Check sheet for the modelled part. Datum: model origin and axes. Units: mm. A direction names the side the tool comes from. Round coordinates to 2 decimals unless told otherwise and drop trailing zeros. Write each loop counter-clockwise with the first axis right and the second up, starting at its lowest first coordinate (ties: lowest second). Pieces come first, ordered by that corner, then holes.
Item 1: Tool access check on faces 1 (the flat face through (24, -8, 20)), 2 (the cylindrical face through (2.994, 22.804, 1.479)), 3 (the flat face through (-11.77, 30.07, 4.93)), 4 (the flat face through (-20.16, 25.23, 4.93)). Record the directions out of +Z, -Z, +X, -X, +Y, -Y that give a thin tool (end or side, any length) a straight path to the whole face; none if there is none.
Item 2: Release check for a two-part mould opening along Z. For faces 5 (the cylindrical face through (-26.6, -0.1, 9.5)), 6 (the cylindrical face through (-13.17, -28.36, 15.07)), 7 (the flat face through (33.5, 0.1, 10)) record: +Z half, -Z half, draft (parallel to the pull), parting line (faces both ways), or undercut.
Item 3: Go/stop test with flat-tipped pins: pin 1 Ø2 at (x, y) = (-26, 25) entering from -Z; pin 2 Ø12 at (x, z) = (10.5, 13.5) entering from -Y; pin 3 Ø6 at (y, z) = (-18, 16) entering from +X; pin 4 Ø5 at (y, z) = (-6.5, 15) entering from +X. Record where each tip stops, or that it passes through.
Item 4: Cross-section at D-D on x = -27. Enter the section's corners in (y, z), plus the area to 3 significant figures.
Item 5: Cross-section at B-B on z = 12. Enter the section's corners in (x, y).
Item 6: Cross-section at C-C on y = 0. Count the separate pieces of the cut face and the enclosed holes in it, plus the area to 3 significant figures.
Item 7: Material ranges on line 1 (X direction, y = 0, z = 0.85); line 2 (Y direction, x = 0, z = 13); line 3 (Y direction, x = 0, z = 1.6), recorded low to high.
Autodesk Inventor part; units mm, degrees
ref_plane "Arbeitsebene1" through (-40, 0, 0) normal (1, 0, 0) x (0, 1, 0)
ref_plane "XZ Plane" through (0, 0, 0) normal (0, 1, 0) x (-1, 0, 0)
ref_plane "XY Plane" through (0, 0, 0) normal (0, 0, 1) x (1, 0, 0)
sketch "Skizze1" plane through (0, 0, 0) normal (0, 1, 0) x (-1, 0, 0)
  line L0 (17, 30.75) -> (17, 26.75)
  line L1 (17, 26.75) -> (20, 26.75)
  line L2 (20, 26.75) -> (20, 6.75)
  line L3 (23, 0) -> (35, 0)
  line L4 (35, 0) -> (35, 20)
  line L5 (35, 20) -> (25, 20)
  line L6 (25, 20) -> (25, 30.75)
  line L7 (17, 30.75) -> (25, 30.75)
  line L8 (0, 0) -> (0, 48.4152)
  line L9 (20, 6.75) -> (23, 6.75)
  line L10 (23, 6.75) -> (23, 4.75)
  line L11 (23, 4.75) -> (25, 4.75)
  line L12 (25, 4.75) -> (25, 3)
  line L13 (25, 3) -> (23, 3)
  line L14 (23, 3) -> (23, 0)
  point P0 (17, 4)
  dimension "d1" = 40
  dimension "d3" = 20
  dimension "d4" = 70
  dimension "d5" = 50
  dimension "d7" = 4
  dimension "d10" = 2
  dimension "d11" = 1.75
  dimension "d12" = 3
  dimension "d13" = 3
  dimension "d14" = 2
  dimension "d15" = 34
  dimension "d16" = 20
revolve "Umdrehung1" add sketch "Skizze1" angle 360 about axis through (0, 0, 0) along (0, 0, 1)
sketch "Skizze2" plane through (0, 0, 0) normal (0, 0, -1) x (-1, 0, 0)
  circle A0 centre (0, 0) radius 23
  circle A1 centre (0, 0) radius 35
  arc A2 (-29.325, -4.4491) -> (-29.325, 4.4491) centre (-30, 0) ccw
  line L0 (-29.325, 4.4491) -> (-34.604, 5.25)
  line L1 (-29.325, -4.4491) -> (-34.604, -5.25)
  line L2 (49, 0) -> (-49, 0)
  line L3 (10.8095, -27.6207) -> (12.7554, -32.593)
  arc A3 (18.5155, -23.1717) -> (10.8095, -27.6207) centre (15, -25.9808) ccw
  line L4 (18.5155, -23.1717) -> (21.8486, -27.343)
  line L5 (18.5155, 23.1717) -> (21.8486, 27.343)
  arc A4 (10.8095, 27.6207) -> (18.5155, 23.1717) centre (15, 25.9808) ccw
  line L6 (10.8095, 27.6207) -> (12.7554, 32.593)
  arc A5 (21.8486, 27.343) -> (12.7554, 32.593) centre (0, 0) ccw
  arc A6 (12.7554, -32.593) -> (21.8486, -27.343) centre (0, 0) ccw
  arc A7 (-34.604, 5.25) -> (-34.604, -5.25) centre (0, 0) ccw
  dimension "d17" = 30
  dimension "d18" = 4.5
  dimension "d21" = 360
extrude "Extrusion1" cut sketch "Skizze2" against normal blind 10 contours L2 A1 L0 A2 | A2 L1 A1 L2 | L5 A4 L6 A1 | A1 L3 A3 L4
sketch "Skizze3" plane through (0, 0, 0) normal (0, 0, -1) x (-1, 0, 0)
  arc A0 (10.8095, 27.6207) -> (18.5155, 23.1717) centre (15, 25.9808) ccw
  arc A1 (-29.325, -4.4491) -> (-29.325, 4.4491) centre (-30, 0) ccw
  arc A2 (18.5155, -23.1717) -> (10.8095, -27.6207) centre (15, -25.9808) ccw
  point P0 (-30, 0)
  point P1 (15, 25.9808)
  point P2 (15, -25.9808)
hole "Bohrung1" at (30, 0, 0) at (-15, 25.9808, 0) at (-15, -25.9808, 0) direction (0, 0, 1) diameter 6 end through all
ref_plane "Arbeitsebene1" through (-40, 0, 0) normal (1, 0, 0) x (0, 1, 0)
sketch "Skizze4" plane through (-40, 0, 0) normal (1, 0, 0) x (0, 1, 0)
  line L0 (-25, 20) -> (25, 20)
  line L1 (10, 20) -> (-10, 20)
  line L2 (-10, 20) -> (-10, 0)
  line L3 (-10, 0) -> (10, 0)
  line L4 (10, 0) -> (10, 20)
  line L5 (-27.343, 0) -> (27.343, 0)
  line L6 (0, -4) -> (0, 24)
  point P0 (0, 0)
extrude "Extrusion2" cut sketch "Skizze4" along normal blind 6.4
sketch "Skizze5" plane through (-33.6, 0, 0) normal (-1, 0, 0) x (0, 0, 1)
  line L0 (-6.15, 0) -> (36.9, 0)
  line L1 (0, -9.8) -> (0, 9.8)
  point P0 (0, 0)
  point P1 (12, 0)
  dimension "d47" = 12
hole "Bohrung2" at (-33.6, 0, 12) direction (1, 0, 0) diameter 5 depth 20 tip angle 118
thread "Gewinde1"
chamfer "Fase1" distance 1 angle 45 1 edges at (25, 0, 30.75)
properties part number "KON_Nietmaschine_Deckel" material "Stahl"
Response values:
1. face 1: +Z
1. face 2: -Z
1. face 3: -Z, -X
1. face 4: -Z, +Y
2. face 5: undercut
2. face 6: draft
2. face 7: -Z half
3. pin 1: passes through
3. pin 2: stops at y = -34.71
3. pin 3: stops at x = 31.62
3. pin 4: stops at x = 34.77
4. outline: (-22.27, 0) - (22.27, 0) - (22.27, 20) - (-22.27, 20) - close; hole circle Ø5 at (0, 12)
4. area: 871 mm2
5. outline: (-33.6, -9.8) arc R35 ccw (long way) to (-33.6, 9.8) - (-33.6, 2.5) - (-19.84, 2.5) arc R20 cw (long way) to (-19.84, -2.5) - (-33.6, -2.5) - close; hole circle Ø6 at (-15, -25.98); hole circle Ø6 at (-15, 25.98); hole circle Ø6 at (30, 0)
6. separate pieces: 4
6. enclosed holes: 0
6. area: 432 mm2
7. line 1: x = -33.6 to -23, 23 to 25.5
7. line 2: y = -35 to -20, 20 to 35
7. line 3: y = -35 to -23, 23 to 35
